CAD build for the part. Positions are in the model's coordinates, mm. A direction names the side the tool comes from. Give positions to 0.01 mm unless a question says otherwise; leave off trailing zeros. Order: outer loops, then holes, each group sorted by start corner. A loop starts at its lowest first (then second) coordinate and runs counter-clockwise, first axis right, second up. Notation, with made-up numbers: M -5,0 L 6,0 A11 ccw 6,7 Z; hole C -35.75,16.5 d5. An arc over 180 degrees is marked long. Put each result on its own line as item: value. Start each with the question number.
1) Drill centre lines: line 1 (Z direction, x = -1, y = 1.25); line 2 (Z direction, x = -5.75, y = -7.5); line 3 (Y direction, x = 3, z = 2.5). Where is each one in solid material? Low to high. Write a range as [from, to].
2) Cut at B-B (y = -0.75). Write the cut outline in (x, z), and give its area (3 significant figures).
3) Cut at C-C (z = 4.5). Write the cut outline in (x, y), and give its area (3 significant figures).
4) Pin check, flat tips, straight feed: pin 1 (5 mm diameter, centred on x = -4.5, z = -0.5, fed in from -Y); pin 2 (0.6 mm diameter, centred on y = -4.5, z = -4.5, fed in from +X); pin 3 (1.8 mm diameter, centred on x = 1, y = -6, fed in from -Z); pin 4 (3 mm diameter, centred on x = -2, z = -3, fed in from +Y). Stop position of each tip, or through.
5) Tool access for faces 1 (the face through (0, 2, -3.5)), 2 (the face through (0, -5, -4.5)), 3 (the face through (0, -1, -3.25)), 4 (the face through (0, 2, -5)): list every direction of +Z, -Z, +X, -X, +Y, -Y with a clear straight run to the whole face (end or side of a thin tool).
6) Cut at A-A (x = -2). Write the cut outline in (y, z), and give its area (3 significant figures).
```python
from build123d import *

# Parameters (mm, degrees)
SKETCH_1_W      = 14
SKETCH_1_H      = 10.5
EXTRUDE_1_DEPTH = 0.9
SKETCH_3_W      = 14
SKETCH_3_H      = 2
EXTRUDE_2_DEPTH = 2
SKETCH_4_W      = 13
SKETCH_4_H      = 0.5
EXTRUDE_3_DEPTH = 6
SKETCH_8_W      = 14
SKETCH_8_H      = 1.5
EXTRUDE_4_DEPTH = 1.5


with BuildPart() as part:
    # Эскиз1 → Бобышка-Вытянуть1 (new body)
    with BuildSketch(Plane(origin=(0, 0, 0), x_dir=(1, 0, 0), z_dir=(0, 1, 0))):
        Rectangle(SKETCH_1_W, SKETCH_1_H)
    extrude(amount=EXTRUDE_1_DEPTH)

    # Эскиз3 → Бобышка-Вытянуть2 (add)
    with BuildSketch(Plane.XZ):
        with Locations((0, -4.25)):
            Rectangle(SKETCH_3_W, SKETCH_3_H)
    extrude(amount=EXTRUDE_2_DEPTH)

    # Эскиз4 → Бобышка-Вытянуть3 (add)
    with BuildSketch(Plane.XZ.offset(2)):
        with Locations((0, -4.25)):
            Rectangle(SKETCH_4_W, SKETCH_4_H)
    extrude(amount=EXTRUDE_3_DEPTH)

    # Эскиз8 → Бобышка-Вытянуть4 (add)
    with BuildSketch(Plane(origin=(0, 0.9, 0), x_dir=(1, 0, 0), z_dir=(0, 1, 0))):
        with Locations((0, 4.25)):
            Rectangle(SKETCH_8_W, SKETCH_8_H)
    extrude(amount=EXTRUDE_4_DEPTH)


solid = part.part
```
Solution:
1. line 1: [-5, -3.5]
1. line 2: [-4.5, -4]
1. line 3: [0, 0.9]
2. outline: M -7,-5.25 L 7,-5.25 L 7,-3.25 L -7,-3.25 Z
2. area: 28.0 mm²
3. outline: M -7,0 L 7,0 L 7,0.9 L -7,0.9 Z
3. area: 12.6 mm²
4. pin 1: y = 0
4. pin 2: x = 6.5
4. pin 3: z = -4.5
4. pin 4: y = 2.4
5. face 1: +Z, +X, -X, +Y
5. face 2: -Z, +X, -X, -Y
5. face 3: +Z, +X, -X, -Y
5. face 4: -Z, +X, -X, +Y
6. outline: M -8,-4.5 L -2,-4.5 L -2,-5.25 L 0.9,-5.25 L 0.9,-5 L 2.4,-5 L 2.4,-3.5 L 0.9,-3.5 L 0.9,5.25 L 0,5.25 L 0,-3.25 L -2,-3.25 L -2,-4 L -8,-4 Z
6. area: 18.7 mm²
